from build123d import *

# Parameters (mm, degrees)
F1_DEPTH      = 3.81
F1_DEPTH_BACK = 7.62
F0_W          = 3.81
F0_H          = 17.78
F2_DEPTH      = 7.62
F3_W          = 17.78
F3_H          = 7.62
F4_DEPTH      = 7.62
F6_DEPTH      = 17.78
F7_W          = 17.78
F7_H          = 11.43
F8_DEPTH      = 33.02
F9_DEPTH      = 17.78
F10_W         = 3.81
F10_H         = 11.43
F11_DEPTH     = 15.24
F12_W         = 3.81
F12_H         = 11.43
F13_DEPTH     = 15.24
F15_DEPTH     = 25.4
F18_DEPTH     = 25.4


# Not quite as in the source:
# - a feature names something its author has since deleted; it is built from what else it names


with BuildPart() as f1:
    # F0 (on Top) → F1 (new body, two sides)
    with BuildSketch(Plane.XY) as f1_sk:
        Polygon((-54.4414605618, -0.1530551207), (-79.8414605618, -0.1530551207), (-79.8414605618, -50.9530551207), (-3.6414605618, -50.9530551207), (-3.6414605618, -0.1530551207), (-29.0414605618, -0.1530551207), (-29.0414605618, -17.9330551207), (-32.8514605618, -17.9330551207), (-32.8514605618, -0.1530551207), (-50.6314605618, -0.1530551207), (-50.6314605618, -17.9330551207), (-54.4414605618, -17.9330551207), align=None)
    extrude(amount=F1_DEPTH)
    extrude(f1_sk.sketch, amount=-F1_DEPTH_BACK)

    # F0 (on Top) → F2 (join)
    with BuildSketch(Plane.XY):
        with Locations((-52.5364605618, -9.0430551207)):
            Rectangle(F0_W, F0_H)
        with Locations((-30.9464605618, -9.0430551207)):
            Rectangle(F0_W, F0_H)
    extrude(amount=-F2_DEPTH)

    # F3 (on face) → F4 (join)
    with BuildSketch(Plane.XY.offset(3.81)):
        with Locations((-41.7414605618, -14.1230551207)):
            Rectangle(F3_W, F3_H)
    extrude(amount=F4_DEPTH)

    # F5 (on face) → F6 (cut)
    with BuildSketch(Plane.YZ.offset(-32.8514605618)):
        Polygon((-14.7124641719, 11.43), (-10.3130551207, 3.81), (-10.3130551207, 11.43), align=None)
        Polygon((-17.9330551207, 9.5705909488), (-14.7124641719, 11.43), (-17.9330551207, 11.43), align=None)
        Polygon((-16.9121686975, 0), (-13.5336460694, 1.9505909488), (-17.9330551207, 9.5705909488), (-17.9330551207, 3.81), (-17.9330551207, 0), align=None)
    extrude(amount=-F6_DEPTH, mode=Mode.SUBTRACT)

    # F7 (on face) → F8 (cut)
    with BuildSketch(Plane.XZ.offset(50.9530551207)):
        with Locations((-41.7414605618, -1.905)):
            Rectangle(F7_W, F7_H)
    extrude(amount=-F8_DEPTH, mode=Mode.SUBTRACT)

    # F9 (add): a face of the model
    f9_faces = [f1.faces().sort_by_distance(p)[0] for p in [
        (-41.7414605618, -0.1530551207, -2.0363793103),
    ]]
    extrude(f9_faces, amount=F9_DEPTH)

    # F10 (on face) → F11 (join)
    with BuildSketch(Plane.XZ.offset(50.9530551207)):
        with Locations((-52.5364605618, -1.905)):
            Rectangle(F10_W, F10_H)
    extrude(amount=F11_DEPTH)

    # F12 (on face) → F13 (join)
    with BuildSketch(Plane.XZ.offset(50.9530551207)):
        with Locations((-30.9464605618, -1.905)):
            Rectangle(F12_W, F12_H)
    extrude(amount=F13_DEPTH)

    # F14 (on face) → F15 (cut)
    with BuildSketch(Plane(origin=(-54.4414605618, 0, 0), x_dir=(0, -1, 0), z_dir=(-1, 0, 0))):
        Polygon((66.1930551207, 3.81), (50.9530551207, 3.81), (66.1930551207, -7.62), align=None)
    extrude(amount=-F15_DEPTH, mode=Mode.SUBTRACT)

    # F16 (on face) + F17 (on face) → F18 (cut)
    with BuildSketch(Plane.XY.offset(3.81)):
        Polygon((-54.4414605618, -50.9530551207), (-72.2214605618, 17.6269448793), (-79.8414605618, 17.6269448793), (-79.8414605618, -50.9530551207), align=None)
    with BuildSketch(Plane.XY.offset(3.81)):
        Polygon((-3.6414605618, 17.6269448793), (-11.2614605618, 17.6269448793), (-29.0414605618, -50.9530551207), (-3.6414605618, -50.9530551207), align=None)
    extrude(amount=-F18_DEPTH, mode=Mode.SUBTRACT)


solid = f1.part
Could you check a few things on this model? Use its own coordinates, in mm. A direction names the side the tool comes from. Coordinates: 2 decimals unless noted, no trailing zeros. Write each loop counter-clockwise with the first axis right and the second up, starting at its lowest first coordinate (ties: lowest second). Pieces come first, ordered by that corner, then holes. Notation, with made-up numbers: (-10, -40) - (10, -40) arc R17 cw to (10, -29) - close; hole circle Ø10 at (76.25, -8.75). An arc over 180 degrees is marked (long way). Write item = value, one per line.
1) We'd pull the mould along Z, two halves only. Please class faces 1 (the flat face through (-41.6, -15.7, 5.7)), 2 (the flat face through (-25, -9, 3.81)), 3 (the flat face through (-42, -17.933, -4)), 4 (the flat face through (-41.62, -15.25, 0.96)): +Z half, -Z half, draft (parallel to the pull), parting line (faces both ways), or undercut.
Result set:
face_1 = undercut
face_2 = +Z half
face_3 = draft
face_4 = undercut
2) Suppose I cut it at C-C on z = -3. Please give me the cut outline in (x, y).
Result set:
outline = (-72.22, 17.63) - (-54.44, -50.95) - (-54.44, -60.03) - (-50.63, -60.03) - (-50.63, -17.93) - (-32.85, -17.93) - (-32.85, -60.03) - (-29.04, -60.03) - (-29.04, -50.95) - (-11.26, 17.63) - close
3) Please list where these lines run through material, in increasing order: line 1 (X direction, y = -56, z = -1); line 2 (X direction, y = -13.5, z = 1.5); line 3 (X direction, y = -27.5, z = 1). Write a range as [from, to].
Result set:
line_1 = [-54.44, -50.63], [-32.85, -29.04]
line_2 = [-64.15, -54.44], [-50.63, -32.85], [-29.04, -19.33]
line_3 = [-60.52, -50.63], [-32.85, -22.96]
4) Suppose I cut it at B-B on y = -29.5. Please give me the cut outline in (x, z).
Result set:
outline = (-60, -7.62) - (-50.63, -7.62) - (-50.63, 3.81) - (-60, 3.81) - close; (-32.85, -7.62) - (-23.48, -7.62) - (-23.48, 3.81) - (-32.85, 3.81) - close
5) Will these pins go through, and if not, where does the flat tip stop? pin 1 Ø3 at (y, z) = (-0.5, 1.5) entering from -X; pin 2 Ø19.5 at (x, y) = (-43, 10) entering from +Z; pin 3 Ø5.5 at (y, z) = (-5.5, 5) entering from +X.
Result set:
pin_1 = -67.91
pin_2 = 3.81
pin_3 = -16.61
6) Suppose I cut it at A-A on x = -49. Please give me the cut outline in (y, z), plus the area to 3 significant figures.
Result set:
outline = (-17.93, -7.62) - (17.63, -7.62) - (17.63, 3.81) - (-10.31, 3.81) - (-14.71, 11.43) - (-17.93, 9.57) - (-13.53, 1.95) - (-16.91, 0) - (-17.93, 0) - close
area = 423 mm2
7) For faces 5 (the flat face through (-50.631, -36, -2)), 6 (the flat face through (-54.441, -57, -3)), 7 (the flat face through (-42, 17.627, -2)), 8 (the flat face through (-31, -17.933, 2)), 9 (the flat face through (-30.973, -58.466, -1.825)), which set-ups out of +Z, -Z, +X, -X, +Y, -Y let a thin tool reach every point of the face, with its end or its side?
Result set:
face_5 = +Z, -Z, -Y
face_6 = +Z, -Z, -X, -Y
face_7 = +Z, -Z, +X, -X, +Y
face_8 = +Z, +Y
face_9 = +Z, +X, -X, -Y
8) Suppose I cut it at D-D on y = 7. Please give me the cut outline in (x, z), plus the area to 3 significant figures.
Result set:
outline = (-69.47, -7.62) - (-14.02, -7.62) - (-14.02, 3.81) - (-29.04, 3.81) - (-29.04, 0) - (-32.85, 0) - (-32.85, 3.81) - (-50.63, 3.81) - (-50.63, 0) - (-54.44, 0) - (-54.44, 3.81) - (-69.47, 3.81) - close
area = 605 mm2
